Source: CAD feature listing. Evaluate the final solid. Frame: model axes, mm. A direction names the side the tool comes from. Give positions to 0.01 mm unless a question says otherwise; leave off trailing zeros. Order: outer loops, then holes, each group sorted by start corner. A loop starts at its lowest first (then second) coordinate and runs counter-clockwise, first axis right, second up. Notation, with made-up numbers: M -6.75,6 L 15.25,6 A21 ccw 15.25,40 Z; hole C 32.5,67.25 d7. An arc over 180 degrees is marked long. Use CSV: the item, a comma, the result in double quotes. Start each with the question number.
1. Line query: line 1 along Y through (x, z) = (45, 1.8); line 2 along X through (y, z) = (-146.5, 0.4); line 3 along Y through (x, z) = (161.5, 3.6). Output: solid intervals per line, ascending. Write a range as [from, to].
2. Pin query (flat end, axial travel): P1, Ø1, axis at x = 182.5, y = -118.5, coming from the -Z side; P2, Ø1, axis at x = -23, z = 0.5, coming from the -Y side. Return the tip coordinate at first contact, or that it passes through.
3. Section query B-B, the plane x = 16.5. Return the cut outline in (y, z).
4. Section query A-A, the plane z = 2.25. Return the cut outline in (x, y), plus the area to 3 significant figures.
5. Mould query, pull axis X, two halves, no side actions, for faces 1 (the flat face through (-4, 2, 0)), 2 (the flat face through (-163.33, -150.115, 1.972)). Classes: released by +X, released by -X, zero draft, split by the parting line, or undercut.
6. Reachability of faces 3 (the flat face through (-4, 2, 4)), 4 (the flat face through (163.127, -149.885, 1.972)) from +Z, -Z, +X, -X, +Y, -Y: full face, straight path, thin tool, end or side. Return the list, or none.
from build123d import *

# Parameters (mm, degrees)
BOSS_EXTRUDE1_DEPTH = 4


with BuildPart() as part:
    # Sketch1 → Boss-Extrude1 (new body)
    with BuildSketch(Plane.XY):
        with BuildLine():
            Line((-170.485837704, -158.228756555), (-155.971675407, -141.771243445))
            ThreePointArc((-155.971675407, -141.771243445), (-149.200431962, -136.771243445), (-140.971675407, -135))
            Line((-140.971675407, -135), (140.971675407, -135))
            ThreePointArc((140.971675407, -135), (149.200431962, -136.771243445), (155.971675407, -141.771243445))
            Line((155.971675407, -141.771243445), (170.485837704, -158.228756555))
            ThreePointArc((170.485837704, -158.228756555), (177.257081148, -163.228756555), (185.485837704, -165))
            Line((185.485837704, -165), (258, -165))
            Line((258, -165), (258, 165))
            Line((258, 165), (-258, 165))
            Line((-258, 165), (-258, -165))
            Line((-258, -165), (-185.485837704, -165))
            ThreePointArc((-185.485837704, -165), (-177.257081148, -163.228756555), (-170.485837704, -158.228756555))
        make_face()
    extrude(amount=BOSS_EXTRUDE1_DEPTH)


solid = part.part
Result set:
1,line 1,"[-135, 165]"
1,line 2,"[-258, -160.14], [160.14, 258]"
1,line 3,"[-148.04, 165]"
2,P1,"z = 0"
2,P2,"y = -135"
3,outline,"M -135,0 L 165,0 L 165,4 L -135,4 Z"
4,outline,"M -258,-165 L -185.49,-165 A20 ccw -170.49,-158.23 L -155.97,-141.77 A20 cw -140.97,-135 L 140.97,-135 A20 cw 155.97,-141.77 L 170.49,-158.23 A20 ccw 185.49,-165 L 258,-165 L 258,165 L -258,165 Z"
4,area,"160,000 mm2"
5,face 1,"zero draft"
5,face 2,"undercut"
6,face 3,"+Z, +X, -X, +Y, -Y"
6,face 4,"+Z, -Z, -Y"
